Read the model definition and answer for the solid it produces. Units are mm, in the model's axes. Face numbers are marked on the shaded views. A direction names the side the tool comes from. Coordinates: 2 decimals unless noted, no trailing zeros. Write each loop counter-clockwise with the first axis right and the second up, starting at its lowest first coordinate (ties: lowest second). Pieces come first, ordered by that corner, then holes. Notation, with made-up numbers: (-33.5, 25) -> (-1.5, 25) arc R15 cw to (-1.5, 29) -> close; hole circle Ø3 at (70, 84.25). An arc over 180 degrees is marked (long way). Use CSV: the item, a comma, the result in double quotes.
from build123d import *

# Parameters (mm, degrees)
F0_R     = 3.4544
F0_R_2   = 2.9464
F1_DEPTH = 4.445
F2_DEPTH = 1.905
F3_R     = 1.905
F4_DEPTH = 2.54
F5_R     = 2.54


with BuildPart() as f1:
    # F0 (on Top) → F1 (new body)
    with BuildSketch(Plane.XY):
        Circle(F0_R)
        Circle(F0_R_2, mode=Mode.SUBTRACT)
    extrude(amount=F1_DEPTH)

    # F0 (on Top) → F2 (join)
    with BuildSketch(Plane.XY):
        Circle(F0_R)
        Circle(F0_R_2, mode=Mode.SUBTRACT)
        Circle(F0_R_2)
    extrude(amount=F2_DEPTH)

    # F3 (on face) → F4 (join)
    with BuildSketch(Plane.XY.offset(1.905)):
        Circle(F3_R)
    extrude(amount=F4_DEPTH)

    # F5
    f5_edges = [f1.edges().sort_by_distance(p)[0] for p in [
        (-3.4544, 0, 0),
    ]]
    fillet(f5_edges, radius=F5_R)


solid = f1.part
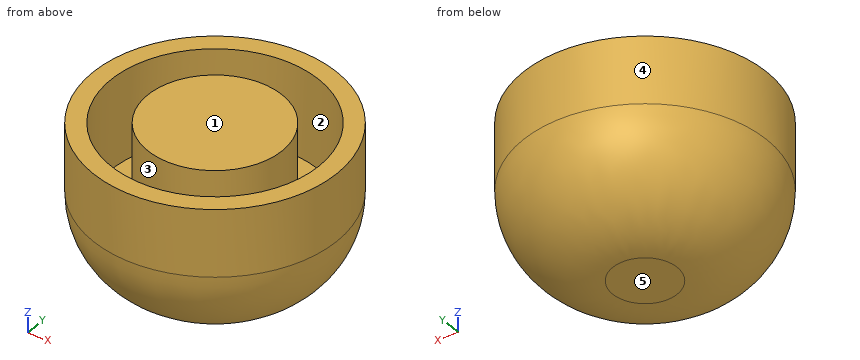
1. A cutting plane is placed at B-B (z = 2.3). Give the number of separate pieces and of enclosed holes in the cut face, and give its area (3 significant figures).
Solutions:
separate pieces,"2"
enclosed holes,"1"
area,"21.4 mm^2"
2. This flat-tipped pin is pushed along its axis until it touches: pin 1 Ø1 at (y, z) = (-1.5, 3.5) entering from -X. Where does it stop, or does it pass through?
Solutions:
pin 1,"stops at x = -3.31"
3. For a pull along X with two mould halves and no side action, classify the marked faces 3, 4 and 5 as pulls with the +X half, pulls with the -X half, needs draft (parallel to the pull), parting line crosses it, or undercut.
Solutions:
face 3,"undercut"
face 4,"parting line crosses it"
face 5,"needs draft"
4. Find the intervals of material crossed by line 1 along Y through (x, z) = (0, 2.85) (3 decimals); line 2 along X through (y, z) = (-0.5, 3); line 3 along Y through (x, z) = (1.5, 2.8), in increasing order.
Solutions:
line 1,"y = -3.454 to -2.946, -1.905 to 1.905, 2.946 to 3.454"
line 2,"x = -3.42 to -2.9, -1.84 to 1.84, 2.9 to 3.42"
line 3,"y = -3.11 to -2.54, -1.17 to 1.17, 2.54 to 3.11"
5. A cutting plane is placed at A-A (z = 3.05). Give the vertices of the cut face in (x, y) (3 decimals), and give its area (3 significant figures).
Solutions:
outline,"circle Ø6.909 at (0, 0); circle Ø3.81 at (0, 0); hole circle Ø5.893 at (0, 0)"
area,"21.6 mm^2"
6. A tool of negligible diameter and unlimited length cuts with its end or side. For the marked faces 1 and 2, from which of +Z, -Z, +X, -X, +Y, -Y can it reach the whole face along a straight path? Write none if from no direction.
Solutions:
face 1,"+Z, +X, -X, +Y, -Y"
face 2,"+Z"
